Could you check a few things on this model? Use its own coordinates, in mm. A direction names the side the tool comes from. Give positions to 0.01 mm unless a question says otherwise; leave off trailing zeros. Order: outer loops, then holes, each group sorted by start corner. A loop starts at its lowest first (then second) coordinate and runs counter-clockwise, first axis right, second up.
(1) If I drill on probe 1 along Z at (x, y) = (3, 0); probe 2 along Z at (x, y) = (-0.5, -0.5); probe 3 along Y at (x, z) = (1.5, 8.75), over which ranges is the centre line in solid material (lowest first)?
(2) Imagine slicing it at B-B, the plane z = 3. Write out the boundary of the cut face in (x, y).
(3) If we mould it in two halves opening along X, with no side actions, what happens to faces 1 (the flat face through (-0.587, 1.036, 0.587)), 2 (the cylindrical face through (2.302, 0.725, 6.009)), 3 (the flat face through (2, 0, 0))? For each: released by +X, released by -X, zero draft, split by the parting line, or undercut.
(4) Will these pins go through, and if not, where does the flat tip stop? pin 1 (1.5 mm diameter, centred on y = 0.5, z = 2, fed in from -X); pin 2 (3 mm diameter, centred on y = -3, z = 6.5, fed in from +X); pin 3 (1 mm diameter, centred on y = 0.5, z = 4.5, fed in from -X); pin 4 (3 mm diameter, centred on x = 0.5, z = 1.5, fed in from -Y).
(5) Imagine slicing it at A-A, the plane y = 0. Write out the boundary of the cut face in (x, z), then the cut area to 3 significant figures.
(6) On a 3-axis mill with a long thin cutter (end or side, diameter ignored), from which of +Z, -Z, +X, -X, +Y, -Y can I reach the whole of each face in a straight line? I mean faces 4 (the flat face through (1.191, 0, 1)), 5 (the flat face through (0, 0, 11.112)). Say none if no direction works.
from build123d import *

# Parameters (mm, degrees)
SKETCH1_R          = 2.413
EXTRUDE1_DEPTH     = 11.1125
SKETCH6_R          = 3.96875
EXTRUDE2_DEPTH     = 1.5875
CUT_EXTRUDE1_DEPTH = 1.190625
SKETCH8_R          = 1.374815329
CUT_EXTRUDE2_DEPTH = 1.190625
CUT_EXTRUDE2_TAPER = 45
CHAMFER1_SIZE      = 0.396875


with BuildPart() as part:
    # Sketch1 → Extrude1 (new body)
    with BuildSketch(Plane.XY):
        Circle(SKETCH1_R)
    extrude(amount=EXTRUDE1_DEPTH)

    # Sketch4 → Cut-Revolve1 (revolve, cut)
    with BuildSketch(Plane(origin=(0, 0, 0), x_dir=(0, 0, -1), z_dir=(1, 0, 0))):
        Polygon((-10.556710267, 2.413), (-11.1125, 1.61925), (-11.1125, 2.413), align=None)
    revolve(axis=Axis((0, 0, 0), (0, 0, 1)), mode=Mode.SUBTRACT)

    # Sketch6 → Extrude2 (add)
    with BuildSketch(Plane.XY):
        Circle(SKETCH6_R)
    extrude(amount=EXTRUDE2_DEPTH)

    # Sketch7 → Cut-Extrude1 (cut)
    with BuildSketch(Plane.XY):
        Polygon((0, 1.374815329), (-1.190625, 0.687407664), (-1.190625, -0.687407664), (0, -1.374815329), (1.190625, -0.687407664), (1.190625, 0.687407664), align=None)
    extrude(amount=CUT_EXTRUDE1_DEPTH, mode=Mode.SUBTRACT)

    # Sketch8 → Cut-Extrude2 (cut)
    with BuildSketch(Plane.XY):
        Circle(SKETCH8_R)
    extrude(amount=CUT_EXTRUDE2_DEPTH, taper=CUT_EXTRUDE2_TAPER, mode=Mode.SUBTRACT)

    # Chamfer1
    chamfer1_edges = [part.edges().sort_by_distance(p)[0] for p in [
        (-3.96875, 0, 1.5875),
        (-3.96875, 0, 0),
    ]]
    chamfer(chamfer1_edges, length=CHAMFER1_SIZE)


solid = part.part
Answer block:
1. probe 1: z = 0 to 1.59
1. probe 2: z = 1.19 to 11.11
1. probe 3: y = -1.89 to 1.89
2. outline: circle Ø4.83 at (0, 0)
3. face 1: undercut
3. face 2: split by the parting line
3. face 3: zero draft
4. pin 1: stops at x = -3.88
4. pin 2: stops at x = 1.89
4. pin 3: stops at x = -2.41
4. pin 4: stops at y = -3.97
5. outline: (-3.97, 0.4) - (-3.57, 0) - (-1.37, 0) - (-1.19, 0.18) - (-1.19, 1.19) - (1.19, 1.19) - (1.19, 0.18) - (1.37, 0) - (3.57, 0) - (3.97, 0.4) - (3.97, 1.19) - (3.57, 1.59) - (2.41, 1.59) - (2.41, 10.56) - (1.62, 11.11) - (-1.62, 11.11) - (-2.41, 10.56) - (-2.41, 1.59) - (-3.57, 1.59) - (-3.97, 1.19) - close
5. area: 54.9 mm2
6. face 4: -Z
6. face 5: +Z, +X, -X, +Y, -Y
